Drawing for the job (mm, zero at the part's lowest x, y, z). A direction names the side the tool comes from. Give positions to 0.01 mm unless a question says otherwise; leave off trailing zeros. Order: outer loops, then holes, each group sorted by start corner. A loop starts at its lowest first (then second) coordinate and runs counter-clockwise, first axis right, second up. Notation, with made-up numbers: (83.25, 51.5) - (127.25, 51.5) arc R21 ccw to (127.25, 73.5) - close; hole circle Ø2 at (23.5, -19). An arc over 180 degrees is marked (long way). One line per item, written item: value.
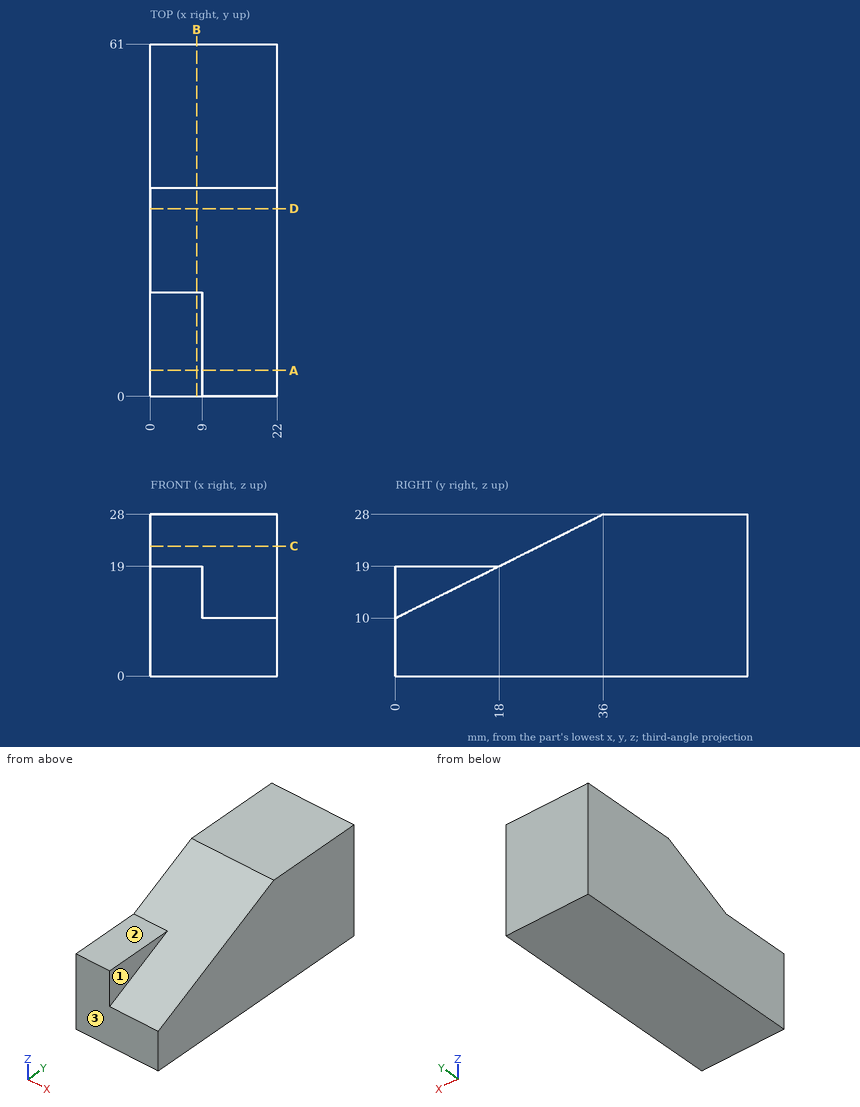
1) Pin check, flat tip, straight feed: pin 1 (4.5 mm diameter, centred on x = 4, y = 9, fed in from +Z). Stop position of the tip, or through.
Outcome:
pin 1: stops at z = 19
2) Drill centre lines: line 1 along Z through (x, y) = (3, 4.5); line 2 along Z through (x, y) = (4.75, 33.5); line 3 along Y through (x, z) = (9, 26). Where is each one in solid material? Low to high. Write a range as from..to.
Outcome:
line 1: z = 0..19
line 2: z = 0..26.75
line 3: y = 32..61
3) Cut at D-D, the plane y = 32.5. Give the cut face in (x, z), then the cut area to 4 significant figures.
Outcome:
outline: (0, 0) - (22, 0) - (22, 26.25) - (0, 26.25) - close
area: 577.5 mm^2
4) Cut at C-C, the plane z = 22.5. Give the cut face in (x, y).
Outcome:
outline: (0, 25) - (22, 25) - (22, 61) - (0, 61) - close
5) Cut at B-B, the plane x = 8. Give the cut face in (y, z).
Outcome:
outline: (0, 0) - (61, 0) - (61, 28) - (36, 28) - (18, 19) - (0, 19) - close
6) Cut at A-A, the plane y = 4.5. Give the cut face in (x, z), then the cut area to 3 significant figures.
Outcome:
outline: (0, 0) - (22, 0) - (22, 12.25) - (9, 12.25) - (9, 19) - (0, 19) - close
area: 330 mm^2
7) Which spindle directions (+Z, -Z, +X, -X, +Y, -Y) get a long thin tool onto all of the face, cutting with end or side? Do the marked faces 1, 2 and 3. Say none if no direction does.
Outcome:
face 1: +Z, +X, -Y
face 2: +Z, +X, -X, -Y
face 3: +Z, -Z, +X, -X, -Y
